For this review, take the finished solid that the model builds, in its own axes (mm). A direction names the side the tool comes from. Give positions to 0.01 mm unless a question says otherwise; leave off trailing zeros. Loops run counter-clockwise (first coordinate to the right, second up) from the corner with the lowest first, then second, coordinate; pieces in that order, holes last.
```python
from build123d import *

# Parameters (mm, degrees)
SKETCH1_R                                        = 101.6
SKETCH1_R_2                                      = 0.254
BOSS_EXTRUDE1_DEPTH                              = 6.35
CBORE_FOR_M5_HEX_HEAD_MACHINE_SCREW1_D           = 5.5
CBORE_FOR_M5_HEX_HEAD_MACHINE_SCREW1_CBORE_D     = 11.71
CBORE_FOR_M5_HEX_HEAD_MACHINE_SCREW1_CBORE_DEPTH = 3.8
CIRPATTERN1_COUNT                                = 12
F_1_8_NPT_TAPPED_HOLE1_AT_2_COUNT                = 2
F_1_8_NPT_TAPPED_HOLE1_AT_2_PITCH                = 68.188989136
F_1_8_NPT_TAPPED_HOLE1_AT_3_COUNT                = 2
F_1_8_NPT_TAPPED_HOLE1_AT_3_PITCH                = 102.325089279
F_1_8_NPT_TAPPED_HOLE1_AT_4_COUNT                = 2
F_1_8_NPT_TAPPED_HOLE1_AT_4_PITCH                = 76.293418173
M10X1_0_TAPPED_HOLE1_D                           = 9
M10X1_0_TAPPED_HOLE1_DEPTH                       = 25.146
M10X1_0_TAPPED_HOLE1_TIP                         = 2.703872786


with BuildPart() as part:
    # Sketch1 → Boss-Extrude1 (new body)
    with BuildSketch(Plane(origin=(0, 0, 0), x_dir=(1, 0, 0), z_dir=(0, 1, 0))):
        with Locations(Location((0, 0, 0), (0, 0, 270))):
            Circle(SKETCH1_R)
        with Locations(Location((-74.964980341, 38.201709762, 0), (0, 0, 270))):
            Circle(SKETCH1_R_2, mode=Mode.SUBTRACT)
    extrude(amount=BOSS_EXTRUDE1_DEPTH)

    # CBORE for M5 Hex Head Machine Screw1 (through all)
    with Locations(Plane(origin=(0, 6.35, 0), x_dir=(1, 0, 0), z_dir=(0, 1, 0))):
        with Locations((-74.964980341, 38.201709762)):
            cbore_for_m5_hex_head_machine_screw1 = CounterBoreHole(CBORE_FOR_M5_HEX_HEAD_MACHINE_SCREW1_D / 2, CBORE_FOR_M5_HEX_HEAD_MACHINE_SCREW1_CBORE_D / 2, CBORE_FOR_M5_HEX_HEAD_MACHINE_SCREW1_CBORE_DEPTH)

    # CirPattern1: CBORE for M5 Hex Head Machine Screw1 ×12 about axis
    cirpattern1_axis = Axis((0, 0, 0), (0, 1, 0))
    for i in range(1, CIRPATTERN1_COUNT):
        add(cbore_for_m5_hex_head_machine_screw1.rotate(cirpattern1_axis, i * 360 / CIRPATTERN1_COUNT), mode=Mode.SUBTRACT)

    # Sketch10 → 1/8 NPT Tapped Hole1 (revolve, cut)
    with BuildSketch(Plane(origin=(-34.094494568, 6.35, -38.146709086), x_dir=(0, 0, 1), z_dir=(1, 0, 0))):
        Polygon((0, 0), (0, 6.35), (4.2164, 6.35), (4.2164, 6.858), (4.936181096, 6.858), (5.1415188, 0), align=None)
    f_1_8_npt_tapped_hole1 = revolve(axis=Axis((-34.094494568, 12.7, -38.146709086), (0, -1, 0)), mode=Mode.SUBTRACT)

    # 1/8 NPT Tapped Hole1 at 2: 1/8 NPT Tapped Hole1 ×2
    with Locations(*[(i * F_1_8_NPT_TAPPED_HOLE1_AT_2_PITCH, 0, 0) for i in range(1, F_1_8_NPT_TAPPED_HOLE1_AT_2_COUNT)]):
        add(f_1_8_npt_tapped_hole1, mode=Mode.SUBTRACT)

    # 1/8 NPT Tapped Hole1 at 3: 1/8 NPT Tapped Hole1 ×2
    with Locations(*[Vector(0.6663955987411356, 0, 0.7455983543292215) * (i * F_1_8_NPT_TAPPED_HOLE1_AT_3_PITCH) for i in range(1, F_1_8_NPT_TAPPED_HOLE1_AT_3_COUNT)]):
        add(f_1_8_npt_tapped_hole1, mode=Mode.SUBTRACT)

    # 1/8 NPT Tapped Hole1 at 4: 1/8 NPT Tapped Hole1 ×2
    with Locations(*[(0, 0, i * F_1_8_NPT_TAPPED_HOLE1_AT_4_PITCH) for i in range(1, F_1_8_NPT_TAPPED_HOLE1_AT_4_COUNT)]):
        add(f_1_8_npt_tapped_hole1, mode=Mode.SUBTRACT)

    # M10x1.0 Tapped Hole1
    with Locations(Plane(origin=(0, 6.35, -31.75), x_dir=(0, 0, 1), z_dir=(0, 1, 0))):
        with Locations((0, 0), (63.331589409, 0)):
            Hole(M10X1_0_TAPPED_HOLE1_D / 2, depth=M10X1_0_TAPPED_HOLE1_DEPTH)
            with Locations((0, 0, -(M10X1_0_TAPPED_HOLE1_DEPTH + M10X1_0_TAPPED_HOLE1_TIP / 2))):  # 118° drill point
                Cone(0, M10X1_0_TAPPED_HOLE1_D / 2, M10X1_0_TAPPED_HOLE1_TIP, mode=Mode.SUBTRACT)


solid = part.part
```
Item 1: For L1, parallel to X at y = 4.75, z = -39; L2, parallel to Z at x = 75.5, y = 5.5; L3, parallel to X at y = 4.25, z = 41.5, list the stretches that pass through material, from the lowest coordinate up.
Answer:
L1: x = -93.82 to -80.77, -69.16 to -39.12, -29.07 to 29.07, 39.12 to 93.82
L2: z = -67.99 to -48.97, -42.67 to 32.37, 44.03 to 67.99
L3: x = -92.74 to -74.52, -66.61 to -37.91, -30.28 to 30.28, 37.91 to 70.13, 79.8 to 92.74
Item 2: Take a section at A-A on y = 4. State how many separate pieces and enclosed holes the cut face has, and give its area (3 significant figures).
Answer:
separate pieces: 1
enclosed holes: 18
area: 30,700 mm2
Item 3: The part is to be moulded in two halves that separate along Z. For faces 1 (the flat face through (-4, 2.55, -81)), 2 (the cylindrical face through (-61.82, 3.13, -80.63)), 3 (the flat face through (1, 0, -1)), say which applies: released by +Z, released by -Z, zero draft, split by the parting line, or undercut.
Answer:
face 1: undercut
face 2: split by the parting line
face 3: zero draft
Item 4: Tool access review of faces 4 (the conical face through (33.87, 3.22, -43.19)), 5 (the cylindrical face through (-77.588, 1.257, -39.028)): name each direction out of +Z, -Z, +X, -X, +Y, -Y from which nothing blocks a thin tool from reaching the whole face with its end or side.
Answer:
face 4: +Y
face 5: +Y, -Y
Item 5: Clearance check with flat-ended pins moving along their axes: pin 1 Ø6 at (x, z) = (-71.5, 46) entering from +Y; pin 2 Ø1.5 at (y, z) = (3, 19.5) entering from +X; pin 3 Ø1 at (y, z) = (4.5, 19.5) entering from -X. State where each tip first meets the part, or that it passes through.
Answer:
pin 1: stops at y = 2.55
pin 2: stops at x = 99.85
pin 3: stops at x = -99.81
Item 6: Take a section at C-C on z = 58.5. Give the boundary of the cut face in (x, y).
Answer:
outline: (-83.07, 0) - (83.07, 0) - (83.07, 6.35) - (-83.07, 6.35) - close
Item 7: Take a section at B-B on z = -19. Give the boundary of the cut face in (x, y), and give its area (3 significant figures).
Answer:
outline: (-99.81, 0) - (99.81, 0) - (99.81, 6.35) - (-99.81, 6.35) - close
area: 1,270 mm2
